The model under review builds one solid part; all positions refer to its coordinate system, in mm. A direction names the side the tool comes from. Round coordinates to 2 decimals unless told otherwise and drop trailing zeros. Write each loop counter-clockwise with the first axis right and the second up, starting at its lowest first coordinate (ties: lowest second). Pieces come first, ordered by that corner, then holes. Notation, with made-up numbers: (-38.5, 5) -> (-34.5, 5) arc R25 ccw to (-34.5, 39) -> close; hole circle Ø6 at (-2.75, 2.5). An arc over 180 degrees is marked (long way). Return JSON: item names as keys, results as strings. Group by question number.
1. Tool access review of faces 4 (the cylindrical face through (20.36, 47.49, 1.52)), 5 (the cylindrical face through (-10.58, 33.52, 1.48)): name each direction out of +Z, -Z, +X, -X, +Y, -Y from which nothing blocks a thin tool from reaching the whole face with its end or side.
2. For line 1 along Y through (x, z) = (14, 1.7); line 2 along Y through (x, z) = (-8.5, 1.8); line 3 along Y through (x, z) = (8, 1.6), list the stretches that pass through material, from the lowest coordinate up. Write a range as from..to.
3. Mouldability with a two-part tool opening along Y and no side actions: class faces 1 (the flat face through (-13.5, 25, 1)), 2 (the flat face through (0, 0, 1)), 3 (the cylindrical face through (-7.893, 61.723, 1.521)) as pulls with the +Y half, pulls with the -Y half, needs draft (parallel to the pull), parting line crosses it, or undercut.
4. Take a section at B-B, the plane x = 6. Write out the cut boundary in (y, z).
5. Take a section at C-C, the plane z = 2.35. Give the number of separate pieces and of enclosed holes in the cut face, then the cut area to 3 significant figures.
6. Take a section at D-D, the plane y = 57.99. Write out the cut boundary in (x, z).
7. Take a section at A-A, the plane y = 47.5. Write out the cut boundary in (x, z), then the cut area to 3 significant figures.
8. Clearance check with a flat-ended pin moving along its axis: P1, Ø1.8, axis at x = -13.5, y = 37.58, coming from the -Z side. State where the tip first meets the part, or that it passes through.
from build123d import *

# Parameters (mm, degrees)
IZIM3_R                     = 1.5
IZIM3_R_2                   = 8.5
Y_KSEKLIK_EKSTR_ZYON1_DEPTH = 3
RADYUS1_R                   = 3


with BuildPart() as part:
    # Çizim3 → Yükseklik-Ekstrüzyon1 (new body)
    with BuildSketch(Plane.XY):
        Polygon((-11, 0), (11, 0), (20.543175205, 17.576342253), (20.543175205, 47.576342253), (8, 62), (-8, 62), (-20.543175205, 47.576342253), (-20.543175205, 17.576342253), align=None)
        with Locations((-6, 4)):
            Circle(IZIM3_R, mode=Mode.SUBTRACT)
        with Locations((6, 4)):
            Circle(IZIM3_R, mode=Mode.SUBTRACT)
        with Locations((-5.25, 57.99)):
            Circle(IZIM3_R, mode=Mode.SUBTRACT)
        with Locations((5.25, 57.99)):
            Circle(IZIM3_R, mode=Mode.SUBTRACT)
        with Locations((-13.5, 37.576342253)):
            Circle(IZIM3_R, mode=Mode.SUBTRACT)
        with Locations((13.5, 37.576342253)):
            Circle(IZIM3_R, mode=Mode.SUBTRACT)
        with Locations((7.573825848, 17.79076532)):
            Circle(IZIM3_R_2, mode=Mode.SUBTRACT)
        with BuildLine():
            Line((-8.730303993, 36.076342253), (8.730303993, 36.076342253))
            ThreePointArc((8.730303993, 36.076342253), (10.541960108, 33.545213379), (13.5, 32.576342253))
            ThreePointArc((13.5, 32.576342253), (15.389824267, 30.686517986), (13.5, 28.796693719))
            ThreePointArc((13.5, 28.796693719), (1.163957554, 28.522195255), (-4.926174152, 17.79076532))
            ThreePointArc((-4.926174152, 17.79076532), (-9.213087076, 13.503852396), (-13.5, 17.79076532))
            Line((-13.5, 17.79076532), (-13.5, 32.576342253))
            ThreePointArc((-13.5, 32.576342253), (-10.541960108, 33.545213379), (-8.730303993, 36.076342253))
        make_face(mode=Mode.SUBTRACT)
        with BuildLine():
            Line((-8.730303993, 39.076342253), (8.730303993, 39.076342253))
            ThreePointArc((8.730303993, 39.076342253), (10.179901517, 41.314917658), (12.574074074, 42.489860461))
            ThreePointArc((12.574074074, 42.489860461), (0, 51.076342253), (-12.574074074, 42.489860461))
            ThreePointArc((-12.574074074, 42.489860461), (-10.179901517, 41.314917658), (-8.730303993, 39.076342253))
        make_face(mode=Mode.SUBTRACT)
    extrude(amount=Y_KSEKLIK_EKSTR_ZYON1_DEPTH)

    # Radyus1
    radyus1_edges = [part.edges().sort_by_distance(p)[0] for p in [
        (-8, 62, 1.5),
        (8, 62, 1.5),
        (20.543175205, 47.576342253, 1.5),
        (20.543175205, 17.576342253, 1.5),
        (-20.543175205, 17.576342253, 1.5),
        (-20.543175205, 47.576342253, 1.5),
    ]]
    fillet(radyus1_edges, radius=RADYUS1_R)


solid = part.part
Output:
{
 "1": {"face 4": "+Z, -Z, +X, +Y", "face 5": "+Z, -Z"},
 "2": {"line 1": "y = 5.53..12.23, 23.35..28.86, 32.51..36.16, 38.99..55.1", "line 2": "y = 0..13.56, 36.08..39.08, 48.06..61.35", "line 3": "y = 0..9.3, 26.28..30.28, 36.08..39.08, 48.45..61.67"},
 "3": {"face 1": "undercut", "face 2": "pulls with the -Y half", "face 3": "pulls with the +Y half"},
 "4": {"outline": "(0, 0) -> (2.5, 0) -> (2.5, 3) -> (0, 3) -> close; (5.5, 0) -> (9.44, 0) -> (9.44, 3) -> (5.5, 3) -> close; (26.14, 0) -> (30.19, 0) -> (30.19, 3) -> (26.14, 3) -> close; (36.08, 0) -> (39.08, 0) -> (39.08, 3) -> (36.08, 3) -> close; (49.67, 0) -> (56.69, 0) -> (56.69, 3) -> (49.67, 3) -> close; (59.29, 0) -> (62, 0) -> (62, 3) -> (59.29, 3) -> close"},
 "5": {"separate pieces": "1", "enclosed holes": "9", "area": "1,390 mm^2"},
 "6": {"outline": "(-11.49, 0) -> (-6.75, 0) -> (-6.75, 3) -> (-11.49, 3) -> close; (-3.75, 0) -> (3.75, 0) -> (3.75, 3) -> (-3.75, 3) -> close; (6.75, 0) -> (11.49, 0) -> (11.49, 3) -> (6.75, 3) -> close"},
 "7": {"outline": "(-20.36, 0) -> (-9.15, 0) -> (-9.15, 3) -> (-20.36, 3) -> close; (9.15, 0) -> (20.36, 0) -> (20.36, 3) -> (9.15, 3) -> close", "area": "67.2 mm^2"},
 "8": {"P1": "passes through"}
}
